Can you work these out from the drawing? Everything is in mm from the part's minimum corner. Round coordinates to 2 decimals unless told otherwise and drop trailing zeros. Loops run counter-clockwise (first coordinate to the right, second up) from the corner with the lowest first, then second, coordinate; pieces in that order, holes last. Notation, with made-up numbers: (68.25, 53.25) - (73.25, 53.25) arc R28 cw to (73.25, 86.25) - close; hole circle Ø11 at (15, -28.75). An arc over 180 degrees is marked (long way). Answer as a JSON object with one key per item and string values. Group by question number.
1) If I drill on line 1 along X through (y, z) = (3.5, 10) (3 decimals); line 2 along X through (y, z) = (9, 11.75), over which ranges is the centre line in solid material (lowest first)? Write a range as [from, to].
2) Will this pin go through, and if not, where does the flat tip stop? P1, Ø3.5, axis at x = 10, z = 10, coming from the +Y side.
3) I want a section at B-B, the plane y = 7.5. Please give me the cut outline in (x, z) (3 decimals), then the cut area to 3 significant figures.
4) I want a section at D-D, the plane z = 19. Please give me the cut outline in (x, y), then the cut area to 3 significant figures.
5) If we mould it in two halves opening along X, with no side actions, what happens to the marked faces 1, 2 and 3? For each: pulls with the +X half, pulls with the -X half, needs draft (parallel to the pull), parting line crosses it, or undercut.
6) I want a section at A-A, the plane z = 10. Please give me the cut outline in (x, y) (3 decimals).
7) I want a section at C-C, the plane x = 9.25. Please give me the cut outline in (y, z), then the cut area to 3 significant figures.
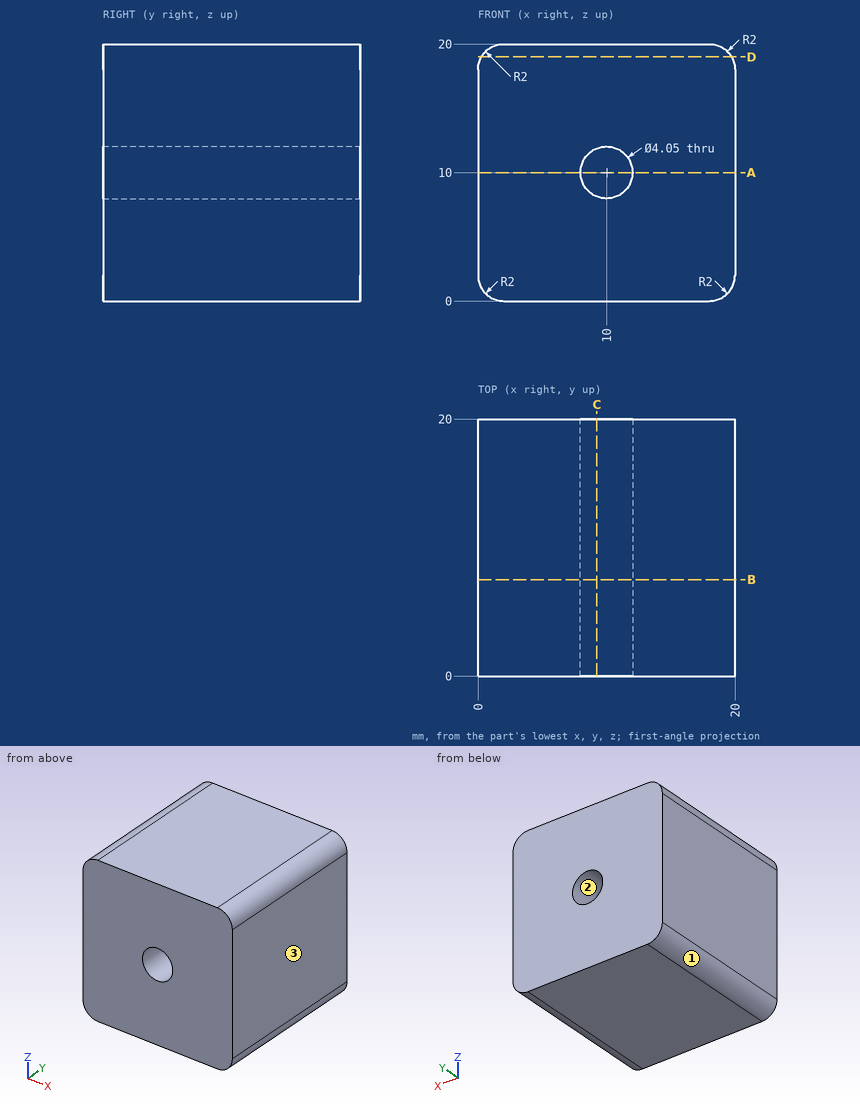
Outcome:
{
 "1": {"line 1": "[0, 7.975], [12.025, 20]", "line 2": "[0, 8.98], [11.02, 20]"},
 "2": {"P1": "through"},
 "3": {"outline": "(0, 2) arc R2 ccw to (2, 0) - (18, 0) arc R2 ccw to (20, 2) - (20, 18) arc R2 ccw to (18, 20) - (2, 20) arc R2 ccw to (0, 18) - close; hole circle Ø4.05 at (10, 10)", "area": "384 mm^2"},
 "4": {"outline": "(0.27, 0) - (19.73, 0) - (19.73, 20) - (0.27, 20) - close", "area": "389 mm^2"},
 "5": {"face 1": "pulls with the -X half", "face 2": "undercut", "face 3": "pulls with the +X half"},
 "6": {"outline": "(0, 0) - (7.975, 0) - (7.975, 20) - (0, 20) - close; (12.025, 0) - (20, 0) - (20, 20) - (12.025, 20) - close"},
 "7": {"outline": "(0, 0) - (20, 0) - (20, 8.12) - (0, 8.12) - close; (0, 11.88) - (20, 11.88) - (20, 20) - (0, 20) - close", "area": "325 mm^2"}
}
